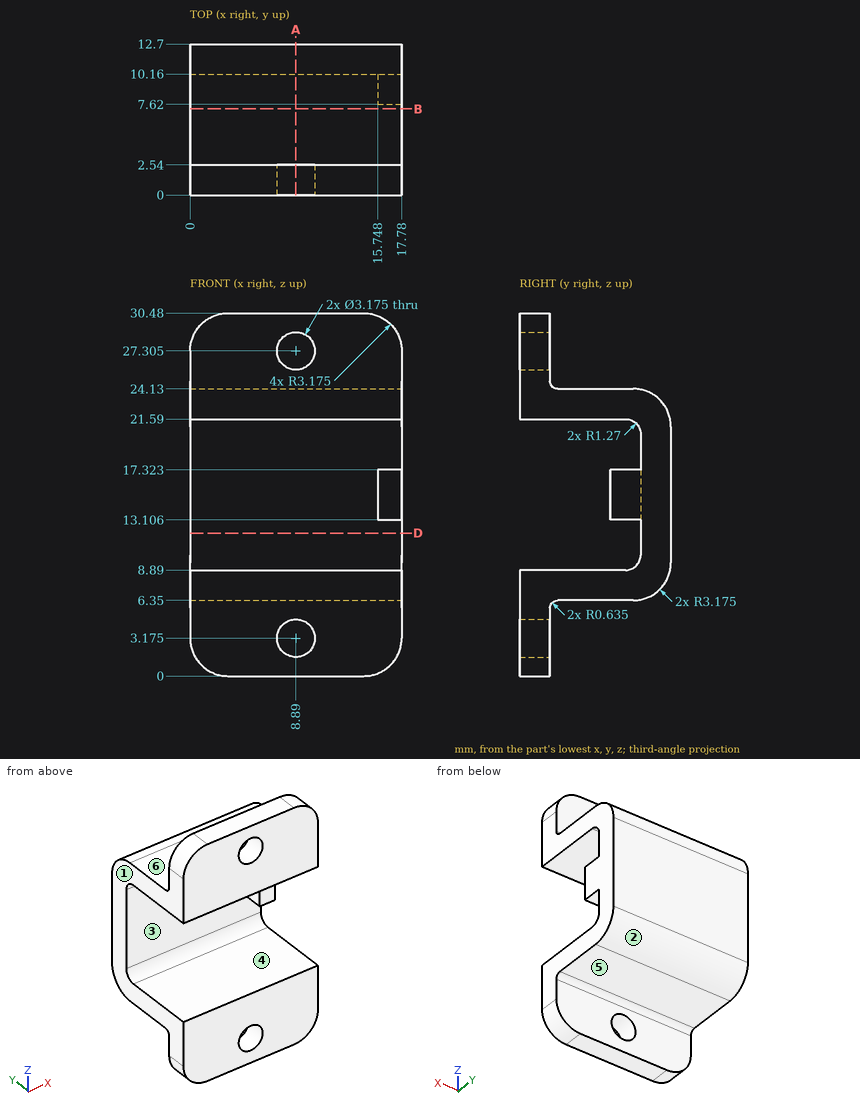
Here's the drawing with two shaded views (mm, measured from the low corner). I have some questions. A direction names the side the tool comes from. Round coordinates to 2 decimals unless told otherwise and drop trailing zeros. Write each loop counter-clockwise with the first axis right and the second up, starting at its lowest first coordinate (ties: lowest second). Pieces come first, ordered by that corner, then holes. Notation, with made-up numbers: M 64,10 L 123,10 A18 cw 123,45 Z; hole C -23,-25 d2. An arc over 180 degrees is marked long. Write each question's results on one line, items separated by ' | '. Start each with the question number.
1. Imagine slicing it at A-A on x = 8.89. Count the separate pieces of the cut face and the enclosed holes in it.
2. Imagine slicing it at B-B on y = 7.25. List the corners of the cut face in (x, z) for me.
3. Imagine slicing it at D-D on z = 12. List the corners of the cut face in (x, y) for me.
4. I need wall thicknesses on L1, parallel to Z at x = 8.89, y = 1.6; L2, parallel to Z at x = 4.75, y = 8.75; L3, parallel to Z at x = 13.25, y = 2.5. Which ranges of each line are inside material? Lowest first, please. Write a range as from..to.
5. On a 3-axis mill with a long thin cutter (end or side, diameter ignored), from which of +Z, -Z, +X, -X, +Y, -Y can I reach the whole of each face in a straight line? I mean the marked faces 4, 5 and 6. Say none if no direction works.
6. I'm going to push flat-ended pins straight in: pin 1 Ø1 at (x, y) = (16.5, 9) entering from +Z; pin 2 Ø1.6 at (x, y) = (16.5, 9) entering from -Z; pin 3 Ø3 at (x, z) = (12.5, 3) entering from +Y. Where does each tip first touch, or does it pass through?
7. Thinking about a two-plate mould opening in Z: for the marked faces 1, 2 and 3, which applies, +Z half, -Z half, draft (parallel to the pull), parting line (faces both ways), or undercut?
Result sheet:
1) separate pieces: 3 | enclosed holes: 0
2) outline: M 0,6.35 L 17.78,6.35 L 17.78,8.89 L 0,8.89 Z; M 0,21.59 L 17.78,21.59 L 17.78,24.13 L 0,24.13 Z
3) outline: M 0,10.16 L 17.78,10.16 L 17.78,12.7 L 0,12.7 Z
4) L1: z = 0..1.59, 4.76..8.89, 21.59..25.72, 28.89..30.48 | L2: z = 6.35..8.89, 21.59..24.13 | L3: z = 0..8.89, 21.59..30.48
5) face 4: +X, -X, -Y | face 5: -Z, +X, -X, +Y | face 6: +Z, +X, -X, +Y
6) pin 1: stops at z = 24.13 | pin 2: stops at z = 6.35 | pin 3: stops at y = 2.54
7) face 1: draft | face 2: -Z half | face 3: undercut
